For this review, take the finished solid that the model builds, in its own axes (mm). A direction names the side the tool comes from. Give positions to 0.01 mm unless a question says otherwise; leave off trailing zeros. Loops run counter-clockwise (first coordinate to the right, second up) from the corner with the lowest first, then second, coordinate; pieces in that order, holes last. Notation, with made-up numbers: M 22,3 L 75,3 A13 ccw 75,12 Z; hole C -8,11.5 d3. An arc over 180 degrees is marked long. Use CSV: the item, a comma, the result in double quotes. Start each with the question number.
1. To check wall thickness, follow line 1 (Z direction, x = -9, y = 7); line 2 (X direction, y = 86.5, z = 86.5) (3 decimals). State the ranges of each line that lie inside material, in increasing order. Write a range as [from, to].
2. Take a section at A-A, the plane z = 94. Write out the cut boundary in (x, y) (3 decimals).
3. The part is to be moulded in two halves that separate along X. For faces 4 (the face through (15.875, 0, -11)), 5 (the face through (0, 12.446, -11)), 6 (the face through (12.446, 0, -11)), 7 (the face through (0, 75, 76.2)), say which applies: pulls with the +X half, pulls with the -X half, needs draft (parallel to the pull), parting line crosses it, or undercut.
4. Insertion check: P1, Ø12.5, axis at x = 0, y = -0.5, coming from the -Z side; P2, Ø2.5, axis at x = -13.5, y = 7.5, coming from the +Z side; P3, Ø6.5, axis at x = 0.5, z = -1.5, coming from the +Y side (3 decimals); P4, Ø3.5, axis at x = 15, y = 2.5, coming from the +Z side. Each pin has a flat end and moves straight along its axis. Give the tip position at first contact, or say it passes through.
5. Tool access review of faces 1 (the face through (0, 15.875, -11)), 2 (the face through (0, -12.446, -11)), 3 (the face through (12.446, 59, 92)): name each direction out of +Z, -Z, +X, -X, +Y, -Y from which nothing blocks a thin tool from reaching the whole face with its end or side.
6. Take a section at B-B, the plane x = -1.5. Write out the cut boundary in (y, z) (3 decimals).
from build123d import *

# Parameters (mm, degrees)
F1_DEPTH      = 76.2
F1_DEPTH_BACK = 101.6
F3_DEPTH      = 152.4


with BuildPart() as f1:
    # F0 (on Top) → F1 (new body, two sides)
    with BuildSketch(Plane.XY) as f1_sk:
        with BuildLine():
            ThreePointArc((15.875, 12.7), (14.945064, 14.945064), (12.7, 15.875))
            Line((12.7, 15.875), (-12.7, 15.875))
            ThreePointArc((-12.7, 15.875), (-14.945064, 14.945064), (-15.875, 12.7))
            Line((-15.875, 12.7), (-15.875, -12.7))
            ThreePointArc((-15.875, -12.7), (-14.945064, -14.945064), (-12.7, -15.875))
            Line((-12.7, -15.875), (12.7, -15.875))
            ThreePointArc((12.7, -15.875), (14.945064, -14.945064), (15.875, -12.7))
            Line((15.875, -12.7), (15.875, 12.7))
        make_face()
        with BuildLine():
            ThreePointArc((10.8585, 12.446), (11.981032, 11.981032), (12.446, 10.8585))
            Line((12.446, 10.8585), (12.446, -10.8585))
            ThreePointArc((12.446, -10.8585), (11.981032, -11.981032), (10.8585, -12.446))
            Line((10.8585, -12.446), (-10.8585, -12.446))
            ThreePointArc((-10.8585, -12.446), (-11.981032, -11.981032), (-12.446, -10.8585))
            Line((-12.446, -10.8585), (-12.446, 10.8585))
            ThreePointArc((-12.446, 10.8585), (-11.981032, 11.981032), (-10.8585, 12.446))
            Line((-10.8585, 12.446), (10.8585, 12.446))
        make_face(mode=Mode.SUBTRACT)
    extrude(amount=F1_DEPTH)
    extrude(f1_sk.sketch, amount=-F1_DEPTH_BACK)

    # F2 (on face) → F3 (join)
    with BuildSketch(Plane.XZ.offset(15.875)):
        with BuildLine():
            Line((-12.7, 76.2), (12.7, 76.2))
            ThreePointArc((12.7, 76.2), (14.945064, 77.129936), (15.875, 79.375))
            Line((15.875, 79.375), (15.875, 104.775))
            ThreePointArc((15.875, 104.775), (14.945064, 107.020064), (12.7, 107.95))
            Line((12.7, 107.95), (-12.7, 107.95))
            ThreePointArc((-12.7, 107.95), (-14.945064, 107.020064), (-15.875, 104.775))
            Line((-15.875, 104.775), (-15.875, 79.375))
            ThreePointArc((-15.875, 79.375), (-14.945064, 77.129936), (-12.7, 76.2))
        make_face()
        with BuildLine():
            Line((-12.446, 81.2165), (-12.446, 102.9335))
            ThreePointArc((-12.446, 102.9335), (-11.981032, 104.056032), (-10.8585, 104.521))
            Line((-10.8585, 104.521), (10.8585, 104.521))
            ThreePointArc((10.8585, 104.521), (11.981032, 104.056032), (12.446, 102.9335))
            Line((12.446, 102.9335), (12.446, 81.2165))
            ThreePointArc((12.446, 81.2165), (11.981032, 80.093968), (10.8585, 79.629))
            Line((10.8585, 79.629), (-10.8585, 79.629))
            ThreePointArc((-10.8585, 79.629), (-11.981032, 80.093968), (-12.446, 81.2165))
        make_face(mode=Mode.SUBTRACT)
    extrude(amount=-F3_DEPTH)


solid = f1.part
Result set:
1,line 1,"[76.2, 79.63], [104.52, 107.95]"
1,line 2,"[-15.875, -12.446], [12.446, 15.875]"
2,outline,"M -15.875,-15.875 L -12.446,-15.875 L -12.446,136.525 L -15.875,136.525 Z; M 12.446,-15.875 L 15.875,-15.875 L 15.875,136.525 L 12.446,136.525 Z"
3,face 4,"pulls with the +X half"
3,face 5,"undercut"
3,face 6,"undercut"
3,face 7,"needs draft"
4,P1,"z = 76.2"
4,P2,"z = 107.95"
4,P3,"y = 15.875"
4,P4,"z = 107.9"
5,face 1,"-Z, +X, -X, +Y"
5,face 2,"-Z"
5,face 3,"+Y, -Y"
6,outline,"M -15.875,-101.6 L -12.446,-101.6 L -12.446,76.2 L 12.446,76.2 L 12.446,-101.6 L 15.875,-101.6 L 15.875,76.2 L 136.525,76.2 L 136.525,79.629 L -15.875,79.629 Z; M -15.875,104.521 L 136.525,104.521 L 136.525,107.95 L -15.875,107.95 Z"
